Input: dimensioned drawing with shaded views. Units: mm. Origin: part minimum x, y, z. A direction names the side the tool comes from. Give positions to 0.01 mm unless a question says otherwise; leave off trailing zeros. Write each loop counter-clockwise with the first axis right and the second up, starting at its lowest first coordinate (ties: lowest second). Pieces come first, ordered by that corner, then holes. Notation, with made-up numbers: (32.25, 34) -> (81.25, 34) arc R26 ccw to (81.25, 72) -> close; hole circle Ø9 at (-10, 19). An arc over 180 degrees is marked (long way). Answer as a JSON object with one key per item and string values.
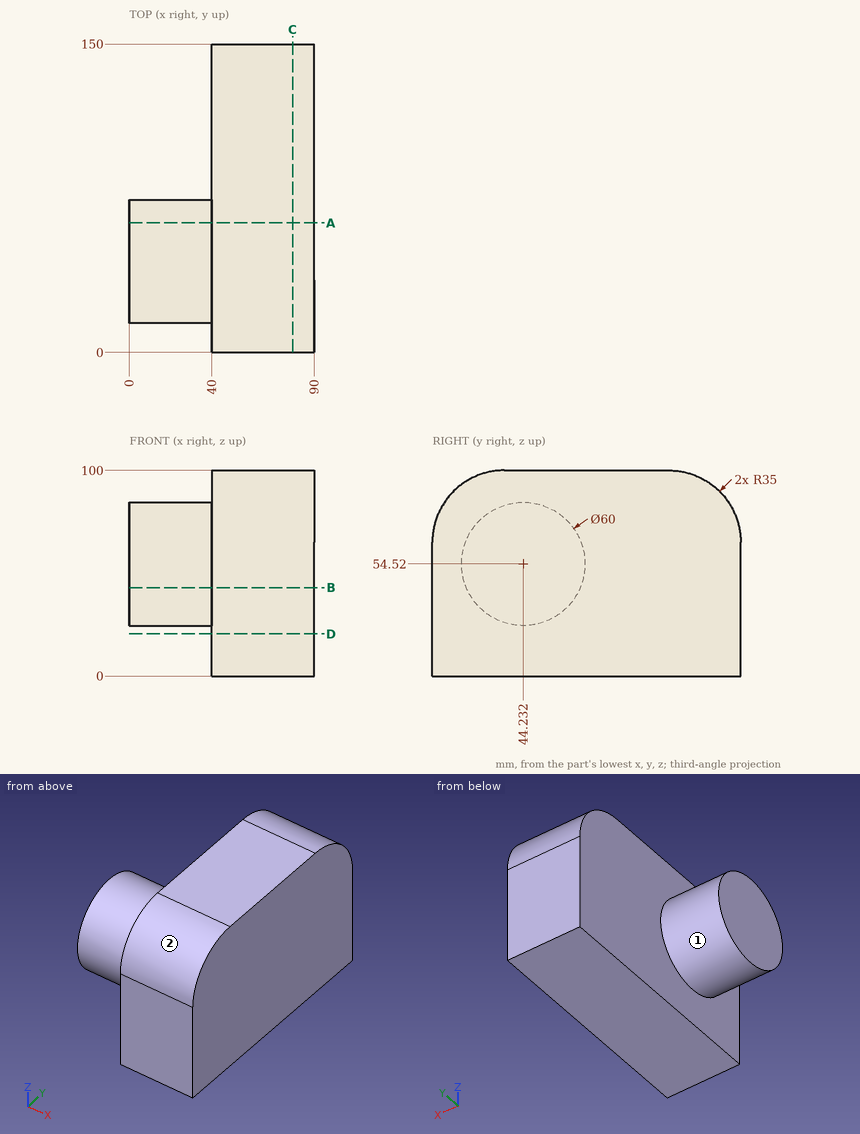
Q1. First-contact query: P1, Ø5, axis at x = 29.5, z = 34, coming from the -Y side; P2, Ø3, axis at x = 44, z = 87.5, coming from the -Y side; P3, Ø4, axis at y = 68, z = 20.5, coming from the -X side; P4, Ø6, axis at x = 54.5, y = 20.5, coming from the -Z side. Flat tips, straight axial feed; report the tip coordinate or a pass-through.
Values:
{"P1": "y = 20.25", "P2": "y = 7", "P3": "x = 40", "P4": "z = 0"}
Q2. Material intervals for L1, parallel to X at y = 81.5, z = 75; L2, parallel to Z at x = 58, y = 25; L3, parallel to Y at x = 58, z = 82.5, sorted ascending. Write a range as from..to.
Values:
{"L1": "40..90", "L2": "0..98.54", "L3": "4.69..145.31"}
Q3. Cut plane B-B (z = 43). Return the cut outline in (x, y), and give its area (3 significant figures).
Values:
{"outline": "(0, 16.53) -> (40, 16.53) -> (40, 0) -> (90, 0) -> (90, 150) -> (40, 150) -> (40, 71.93) -> (0, 71.93) -> close", "area": "9,720 mm²"}
Q4. Cut plane C-C (x = 79.5). Return the cut outline in (y, z).
Values:
{"outline": "(0, 0) -> (150, 0) -> (150, 65) arc R35 ccw to (115, 100) -> (35, 100) arc R35 ccw to (0, 65) -> close"}
Q5. Cut plane A-A (y = 63). Return the cut outline in (x, z) (1 decimal).
Values:
{"outline": "(0, 31.1) -> (40, 31.1) -> (40, 0) -> (90, 0) -> (90, 100) -> (40, 100) -> (40, 77.9) -> (0, 77.9) -> close"}
Q6. Cut plane D-D (z = 20.5). Return the cut outline in (x, y), and give its area (3 significant figures).
Values:
{"outline": "(40, 0) -> (90, 0) -> (90, 150) -> (40, 150) -> close", "area": "7,500 mm²"}
Q7. Set-up query: the marked faces 1 and 2. Return all of +Z, -Z, +X, -X, +Y, -Y with unobstructed straight access to the full face (end or side cutting, diameter ignored); none if empty.
Values:
{"face 1": "-X", "face 2": "+Z, +X, -X, -Y"}
